Can you work these out from the model? Positions are in its coordinate system, mm. A direction names the side the tool comes from. Give positions to 0.01 mm unless a question says otherwise; leave off trailing zeros. Loops run counter-clockwise (first coordinate to the right, second up) from the corner with the lowest first, then second, coordinate; pieces in that order, holes last. Notation, with made-up numbers: M -35.75,49 L -13.75,49 A15 cw -13.75,58 Z; hole C -8.75,19 d7. An arc over 180 degrees is marked long. Answer as a JSON object with one key per item and string values.
```python
from build123d import *

# Parameters (mm, degrees)
F0_W     = 12
F0_H     = 5
F0_W_2   = 5
F0_H_2   = 25
F1_DEPTH = 5


with BuildPart() as f1:
    # F0 (on Right) → F1 (new body)
    with BuildSketch(Plane.YZ):
        Polygon((27.5, 49), (27.5, 69), (20.5, 69), (8.5, 69), (-8.5, 69), (-20.5, 69), (-27.5, 69), (-27.5, 49), (-27.5, 24), (-27.5, -24), (-27.5, -49), (-27.5, -69), (-20.5, -69), (-8.5, -69), (8.5, -69), (20.5, -69), (27.5, -69), (27.5, -49), (27.5, -24), (27.5, 24), align=None)
        with Locations((-14.5, 71.5)):
            Rectangle(F0_W, F0_H)
        with Locations((14.5, 71.5)):
            Rectangle(F0_W, F0_H)
        with Locations((30, 36.5)):
            Rectangle(F0_W_2, F0_H_2)
        with Locations((30, -36.5)):
            Rectangle(F0_W_2, F0_H_2)
        with Locations((14.5, -71.5)):
            Rectangle(F0_W, F0_H)
        with Locations((-14.5, -71.5)):
            Rectangle(F0_W, F0_H)
        with Locations((-30, -36.5)):
            Rectangle(F0_W_2, F0_H_2)
        with Locations((-30, 36.5)):
            Rectangle(F0_W_2, F0_H_2)
    extrude(amount=F1_DEPTH)


solid = f1.part
```
1) If we mould it in two halves opening along Z, with no side actions, what happens to faces 1 (the flat face through (2, -30, 49)), 2 (the flat face through (2, -27.5, 0)), 3 (the flat face through (2, -20.5, -72))? For each: +Z half, -Z half, draft (parallel to the pull), parting line (faces both ways), or undercut.
Answer list:
{"face 1": "+Z half", "face 2": "undercut", "face 3": "draft"}
2) For faces 4 (the flat face through (2, -8.5, 71)), 5 (the flat face through (2, -20.5, 71)), 6 (the flat face through (2, -30, 24)), 7 (the flat face through (2, -8.5, -72)), which set-ups out of +Z, -Z, +X, -X, +Y, -Y let a thin tool reach every point of the face, with its end or its side?
Answer list:
{"face 4": "+Z, +X, -X", "face 5": "+Z, +X, -X, -Y", "face 6": "+X, -X, -Y", "face 7": "-Z, +X, -X"}
3) Suppose I cut it at B-B, the plane y = 6. Write out the boundary of the cut face in (x, z), and give its area (3 significant figures).
Answer list:
{"outline": "M 0,-69 L 5,-69 L 5,69 L 0,69 Z", "area": "690 mm^2"}
4) Suppose I cut it at A-A, the plane z = -14. Write out the boundary of the cut face in (x, y).
Answer list:
{"outline": "M 0,-27.5 L 5,-27.5 L 5,27.5 L 0,27.5 Z"}
5) Will these pins go through, and if not, where does the flat tip stop? pin 1 Ø1.5 at (x, y) = (3, 29) entering from -Z; pin 2 Ø2.5 at (x, z) = (1.5, 4.5) entering from +Y; pin 3 Ø2.5 at (x, z) = (3.5, -71.5) entering from +Y.
Answer list:
{"pin 1": "z = -49", "pin 2": "y = 27.5", "pin 3": "y = 20.5"}
6) Please list where these lines run through material, in increasing order: line 1 along Z through (x, y) = (4.3, -29); line 2 along Y through (x, z) = (2.8, -6); line 3 along Z through (x, y) = (3.1, 4). Write a range as from..to.
Answer list:
{"line 1": "-49..-24, 24..49", "line 2": "-27.5..27.5", "line 3": "-69..69"}
